from build123d import *

# Parameters (mm, degrees)
CROQUIS1_W                 = 30
CROQUIS1_H                 = 30
SALIENTE_EXTRUIR1_DEPTH    = 7
CROQUIS2_W                 = 30
CROQUIS2_H                 = 35
SALIENTE_EXTRUIR2_DEPTH    = 8
CROQUIS3_W                 = 4.85
CROQUIS3_H                 = 35
SALIENTE_EXTRUIR3_DEPTH    = 10
CORTAR_EXTRUIR1_REACH      = 47.804
CROQUIS4_R                 = 2.25
CORTAR_EXTRUIR4_REACH      = 47.804
CROQUIS7_W                 = 30
CROQUIS7_H                 = 30
CROQUIS8_W                 = 15
CROQUIS8_H                 = 4.016004192
SALIENTE_EXTRUIR4_DEPTH    = 30
CORTAR_EXTRUIR5_REACH      = 49.687
CROQUIS9_R                 = 2.25
REDONDEO3_R                = 4
CORTAR_EXTRUIR6_DEPTH      = 55.281880034
CORTAR_EXTRUIR6_DEPTH_BACK = 55.281880034
CROQUIS10_R                = 1.75


with BuildPart() as part:
    # Croquis1 → Saliente-Extruir1 (new body)
    with BuildSketch(Plane.XY):
        Rectangle(CROQUIS1_W, CROQUIS1_H)
    extrude(amount=SALIENTE_EXTRUIR1_DEPTH)

    # Croquis2 → Saliente-Extruir2 (add)
    with BuildSketch(Plane.XZ.offset(15)):
        with Locations((0, 17.5)):
            Rectangle(CROQUIS2_W, CROQUIS2_H)
    extrude(amount=SALIENTE_EXTRUIR2_DEPTH)

    # Croquis3 → Saliente-Extruir3 (add)
    with BuildSketch(Plane(origin=(0, -23, 0), x_dir=(-1, 0, 0), z_dir=(0, -1, 0))):
        with Locations((12.575, -17.5)):
            Rectangle(CROQUIS3_W, CROQUIS3_H)
        with Locations((-12.575, -17.5)):
            Rectangle(CROQUIS3_W, CROQUIS3_H)
    extrude(amount=SALIENTE_EXTRUIR3_DEPTH)

    # Croquis4 → Cortar-Extruir1 (cut, up to next)
    with BuildSketch(Plane.XY.offset(7), mode=Mode.PRIVATE) as cortar_extruir1_sk1:
        with Locations((0, 7)):
            Circle(CROQUIS4_R)
    cortar_extruir1_tool1 = extrude(cortar_extruir1_sk1.sketch, amount=-CORTAR_EXTRUIR1_REACH, mode=Mode.PRIVATE) & part.part
    add(cortar_extruir1_tool1.solids().sort_by_distance((0, 7, 7))[0], mode=Mode.SUBTRACT)

    # Croquis7 → Cortar-Extruir4 (cut, up to next)
    with BuildSketch(Plane.XY.offset(7), mode=Mode.PRIVATE) as cortar_extruir4_sk1:
        Rectangle(CROQUIS7_W, CROQUIS7_H)
    cortar_extruir4_tool1 = extrude(cortar_extruir4_sk1.sketch, amount=-CORTAR_EXTRUIR4_REACH, mode=Mode.PRIVATE) & part.part
    add(cortar_extruir4_tool1.solids().sort_by_distance((0, 0, 7))[0], mode=Mode.SUBTRACT)

    # Croquis8 → Saliente-Extruir4 (add)
    with BuildSketch(Plane(origin=(0, -15, 0), x_dir=(1, 0, 0), z_dir=(0, 1, 0))):
        with Locations((0, -2.008002096)):
            Rectangle(CROQUIS8_W, CROQUIS8_H)
    extrude(amount=SALIENTE_EXTRUIR4_DEPTH)

    # Croquis9 → Cortar-Extruir5 (cut, up to next)
    with BuildSketch(Plane.XY.offset(4.016004192), mode=Mode.PRIVATE) as cortar_extruir5_sk1:
        with Locations((0, 7)):
            Circle(CROQUIS9_R)
    cortar_extruir5_tool1 = extrude(cortar_extruir5_sk1.sketch, amount=-CORTAR_EXTRUIR5_REACH, mode=Mode.PRIVATE) & part.part
    add(cortar_extruir5_tool1.solids().sort_by_distance((0, 7, 4.016004))[0], mode=Mode.SUBTRACT)

    # Redondeo3
    redondeo3_edges = [part.edges().sort_by_distance(p)[0] for p in [
        (7.5, -15, 2.008002096),
        (-7.5, -15, 2.008002096),
        (0, -15, 4.016004192),
    ]]
    fillet(redondeo3_edges, radius=REDONDEO3_R)

    # Croquis10 → Cortar-Extruir6 (cut, two sides: drawn at the far end of the back side and taken through both)
    with BuildSketch(Plane(origin=(-10.15, 0, 0), x_dir=(0, 0, -1), z_dir=(1, 0, 0)).offset(-CORTAR_EXTRUIR6_DEPTH_BACK)):
        with Locations((-10, -28)):
            Circle(CROQUIS10_R)
        with Locations((-25, -28)):
            Circle(CROQUIS10_R)
    extrude(amount=CORTAR_EXTRUIR6_DEPTH + CORTAR_EXTRUIR6_DEPTH_BACK, mode=Mode.SUBTRACT)


solid = part.part
The model under review builds one solid part; all positions refer to its coordinate system, in mm. A direction names the side the tool comes from. Round coordinates to 2 decimals unless told otherwise and drop trailing zeros. Order: outer loops, then holes, each group sorted by start corner. A loop starts at its lowest first (then second) coordinate and runs counter-clockwise, first axis right, second up. Notation, with made-up numbers: (72.5, 23) -> (99.5, 23) arc R16 cw to (99.5, 46) -> close; hole circle Ø8 at (-18, 8.5). An arc over 180 degrees is marked (long way). Write item = value, one per line. Start each with the question number.
Item 1: Consider section B-B on x = 0. Write out the cut boundary in (y, z).
Item 2: Clearance check with flat-ended pins moving along their axes: pin 1 Ø1 at (x, y) = (-5, 5.5) entering from -Z; pin 2 Ø4.5 at (y, z) = (7.5, 1) entering from -X; pin 3 Ø5 at (x, z) = (12, 22.5) entering from +Y; pin 4 Ø8 at (x, z) = (4.5, 24.5) entering from -Y. State where each tip first meets the part, or that it passes through.
Item 3: Mouldability with a two-part tool opening along X and no side actions: class faces 4 (the face through (10.15, -28, 18)), 5 (the face through (0, 2, 4.016)), 6 (the face through (9.24, -14.3, 3.06)) as released by +X, released by -X, zero draft, split by the parting line, or undercut.
Item 4: Consider section D-D on z = 25. Write out the cut boundary in (x, y), plus the area to 3 significant figures.
Item 5: Consider section C-C on y = -28. Write out the cut boundary in (x, z), plus the area to 3 significant figures.
Item 6: For faces 1 (the face through (-10.15, -28, 18)), 2 (the face through (-7.5, 2, 2)), 3 (the face through (15, -24, 17)), list the 3-axis set-ups (+Z, -Z, +X, -X, +Y, -Y) from which the entire face can be reached by the end or side of a thin tool; tool diameter is ignored.
Item 7: For line 1 along Z through (x, y) = (14.05, -28); line 2 along Y through (x, z) = (-13.5, 10); line 3 along Y through (x, z) = (0, 1.65), list the stretches that pass through material, from the lowest coordinate up.
Item 8: Consider section A-A on y = 7. Write out the cut boundary in (x, z), plus the area to 3 significant figures.
Conclusion:
q1.outline = (-23, 0) -> (4.75, 0) -> (4.75, 4.02) -> (-11, 4.02) arc R4 cw to (-15, 8.02) -> (-15, 35) -> (-23, 35) -> close; (9.25, 0) -> (15, 0) -> (15, 4.02) -> (9.25, 4.02) -> close
q2.pin_1 = 0
q2.pin_2 = -7.5
q2.pin_3 = -15
q2.pin_4 = -23
q3.face_4 = undercut
q3.face_5 = zero draft
q3.face_6 = released by +X
q4.outline = (-15, -33) -> (-10.15, -33) -> (-10.15, -29.75) -> (-15, -29.75) -> close; (-15, -26.25) -> (-10.15, -26.25) -> (-10.15, -23) -> (10.15, -23) -> (10.15, -26.25) -> (15, -26.25) -> (15, -15) -> (-15, -15) -> close; (10.15, -33) -> (15, -33) -> (15, -29.75) -> (10.15, -29.75) -> close
q4.area = 303 mm2
q5.outline = (-15, 0) -> (-10.15, 0) -> (-10.15, 8.25) -> (-15, 8.25) -> close; (-15, 11.75) -> (-10.15, 11.75) -> (-10.15, 23.25) -> (-15, 23.25) -> close; (-15, 26.75) -> (-10.15, 26.75) -> (-10.15, 35) -> (-15, 35) -> close; (10.15, 0) -> (15, 0) -> (15, 8.25) -> (10.15, 8.25) -> close; (10.15, 11.75) -> (15, 11.75) -> (15, 23.25) -> (10.15, 23.25) -> close; (10.15, 26.75) -> (15, 26.75) -> (15, 35) -> (10.15, 35) -> close
q5.area = 272 mm2
q6.face_1 = +Z, -Z, -Y
q6.face_2 = +Z, -Z, -X, +Y
q6.face_3 = +Z, -Z, +X, +Y, -Y
q7.line_1 = 0 to 8.25, 11.75 to 23.25, 26.75 to 35
q7.line_2 = -33 to -29.75, -26.25 to -15
q7.line_3 = -23 to 4.75, 9.25 to 15
q8.outline = (-7.5, 0) -> (-2.25, 0) -> (-2.25, 4.02) -> (-7.5, 4.02) -> close; (2.25, 0) -> (7.5, 0) -> (7.5, 4.02) -> (2.25, 4.02) -> close
q8.area = 42.2 mm2
